CAD build for the part. Positions are in the model's coordinates, mm. Face numbers are marked on the shaded views. A direction names the side the tool comes from. Coordinates: 2 decimals unless noted, no trailing zeros. Write each loop counter-clockwise with the first axis right and the second up, starting at its lowest first coordinate (ties: lowest second). Pieces come first, ordered by that corner, then holes. Notation, with made-up numbers: (23, -30) - (29, -30) arc R28 ccw to (29, 2) - close; hole circle Ø11 at (26, 11). An arc over 180 degrees is marked (long way). One line per question, with ' | ' between items. Start each with the question number.
1. Two-plate mould, pull along Z, no slides. Class the marked faces 6, 7, 8 and 9: +Z half, -Z half, draft (parallel to the pull), parting line (faces both ways), or undercut.
2. Probe line 1 (Z direction, x = 0, y = -5); line 2 (Z direction, x = 0, y = -19.5); line 3 (Z direction, x = 0, y = -12.75). List the from-to ranges inside material, lowest first.
3. Band-saw the part on C-C, the plane y = -1.75. Write the cut outline in (x, z), then the cut area to 3 significant figures.
4. Band-saw the part on B-B, the plane y = -20. Write the cut outline in (x, z), then the cut area to 3 significant figures.
5. Band-saw the part on D-D, the plane z = 6. Write the cut outline in (x, y).
6. Flat gauge pins, fed straight in: P1, Ø4, axis at x = 1, y = -22.5, coming from the +Z side; P2, Ø9, axis at y = -5, z = 41.5, coming from the +X side; P3, Ø1.5, axis at x = -3.5, z = 36.5, coming from the -Y side. Where does each tip first touch, or does it go through?
7. Band-saw the part on A-A, the plane x = 0. Write the cut outline in (y, z), then the cut area to 3 significant figures.
8. Which spindle directions (+Z, -Z, +X, -X, +Y, -Y) get a long thin tool onto all of the face, cutting with end or side? Do the marked faces 1, 2, 3, 4 and 5. Say none if no direction does.
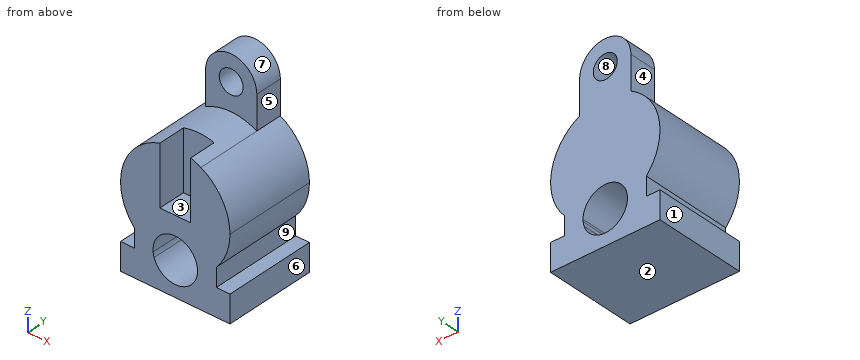
from build123d import *

# Parameters (mm, degrees)
F1_DEPTH = 27
F2_DEPTH = 8
F4_DEPTH = 8


with BuildPart() as f1:
    # F0 (on Front) → F1 (new body)
    with BuildSketch(Plane.XZ):
        with BuildLine():
            ThreePointArc((-7.5, 38.1332940251), (-15.7412312858, 26.8659444529), (-12, 13.4169947557))
            Line((-12, 13.4169947557), (-12, 22))
            Line((-12, 22), (12, 22))
            Line((12, 22), (12, 13.4169947557))
            ThreePointArc((12, 13.4169947557), (14.9666295471, 18.3431457505), (16, 24))
            ThreePointArc((16, 24), (13.7113092008, 32.2462112512), (7.5, 38.1332940251))
            Line((7.5, 38.1332940251), (-7.5, 38.1332940251))
        make_face()
        with BuildLine():
            Line((-12, 22), (-12, 13.4169947557))
            ThreePointArc((-12, 13.4169947557), (-9.454026078, 11.091809154), (-6.4690134152, 9.3660714286))
            ThreePointArc((-6.4690134152, 9.3660714286), (-0.3173427178, 16.4922487321), (6.5, 10))
            ThreePointArc((6.5, 10), (6.4922487321, 9.6826572822), (6.4690134152, 9.3660714286))
            ThreePointArc((6.4690134152, 9.3660714286), (9.454026078, 11.091809154), (12, 13.4169947557))
            Line((12, 13.4169947557), (12, 22))
            Line((12, 22), (-12, 22))
        make_face()
        with BuildLine():
            ThreePointArc((7.5, 38.1332940251), (0, 40), (-7.5, 38.1332940251))
            Line((-7.5, 38.1332940251), (7.5, 38.1332940251))
        make_face()
        with BuildLine():
            Line((-12, 8), (-16, 8))
            Line((-16, 8), (-16, 0))
            Line((-16, 0), (16, 0))
            Line((16, 0), (16, 8))
            Line((16, 8), (12, 8))
            Line((12, 8), (6.1846584384, 8))
            ThreePointArc((6.1846584384, 8), (0, 3.5), (-6.1846584384, 8))
            Line((-6.1846584384, 8), (-12, 8))
        make_face()
        with BuildLine():
            ThreePointArc((6.4690134152, 9.3660714286), (6.3635988742, 8.6753833128), (6.1846584384, 8))
            Line((6.1846584384, 8), (12, 8))
            Line((12, 8), (12, 13.4169947557))
            ThreePointArc((12, 13.4169947557), (9.454026078, 11.091809154), (6.4690134152, 9.3660714286))
        make_face()
        with BuildLine():
            Line((-12, 13.4169947557), (-12, 8))
            Line((-12, 8), (-6.1846584384, 8))
            ThreePointArc((-6.1846584384, 8), (-6.3635988742, 8.6753833128), (-6.4690134152, 9.3660714286))
            ThreePointArc((-6.4690134152, 9.3660714286), (-9.454026078, 11.091809154), (-12, 13.4169947557))
        make_face()
    extrude(amount=F1_DEPTH)

    # F0 (on Front) → F2 (join)
    with BuildSketch(Plane.XZ):
        with BuildLine():
            Line((-3.5, 48), (-7.5, 48))
            ThreePointArc((-7.5, 48), (0, 40.5), (7.5, 48))
            Line((7.5, 48), (3.5, 48))
            ThreePointArc((3.5, 48), (0, 44.5), (-3.5, 48))
        make_face()
        with BuildLine():
            ThreePointArc((7.5, 48), (0, 55.5), (-7.5, 48))
            Line((-7.5, 48), (-3.5, 48))
            ThreePointArc((-3.5, 48), (0, 51.5), (3.5, 48))
            Line((3.5, 48), (7.5, 48))
        make_face()
        with BuildLine():
            Line((-7.5, 48), (-7.5, 38.1332940251))
            ThreePointArc((-7.5, 38.1332940251), (0, 40), (7.5, 38.1332940251))
            Line((7.5, 38.1332940251), (7.5, 48))
            ThreePointArc((7.5, 48), (0, 40.5), (-7.5, 48))
        make_face()
    extrude(amount=F2_DEPTH)

    # F3 (on face) → F4 (cut)
    with BuildSketch(Plane.XZ.offset(27)):
        with BuildLine():
            Line((-4.5, 39.3541525328), (-4.5, 22))
            Line((-4.5, 22), (4.5, 22))
            Line((4.5, 22), (4.5, 39.3541525328))
            ThreePointArc((4.5, 39.3541525328), (0, 40), (-4.5, 39.3541525328))
        make_face()
    extrude(amount=-F4_DEPTH, mode=Mode.SUBTRACT)


solid = f1.part
Filled in:
1) face 6: draft | face 7: +Z half | face 8: undercut | face 9: undercut
2) line 1: z = 0 to 3.5, 16.5 to 44.5, 51.5 to 55.5 | line 2: z = 0 to 3.5, 16.5 to 22 | line 3: z = 0 to 3.5, 16.5 to 40
3) outline: (-16, 0) - (16, 0) - (16, 8) - (12, 8) - (12, 13.42) arc R16 ccw to (7.5, 38.13) - (7.5, 48) arc R7.5 ccw to (-7.5, 48) - (-7.5, 38.13) arc R16 ccw to (-12, 13.42) - (-12, 8) - (-16, 8) - close; hole circle Ø13 at (0, 10); hole circle Ø7 at (0, 48) | area: 1,150 mm²
4) outline: (-16, 0) - (16, 0) - (16, 8) - (12, 8) - (12, 13.42) arc R16 ccw to (4.5, 39.35) - (4.5, 22) - (-4.5, 22) - (-4.5, 39.35) arc R16 ccw to (-12, 13.42) - (-12, 8) - (-16, 8) - close; hole circle Ø13 at (0, 10) | area: 807 mm²
5) outline: (-16, -27) - (-5.12, -27) - (-5.12, 0) - (-16, 0) - close; (5.12, -27) - (16, -27) - (16, 0) - (5.12, 0) - close
6) P1: stops at z = 22 | P2: stops at x = 9.33 | P3: stops at y = -19
7) outline: (-27, 0) - (0, 0) - (0, 3.5) - (-27, 3.5) - close; (-27, 16.5) - (0, 16.5) - (0, 44.5) - (-8, 44.5) - (-8, 40) - (-19, 40) - (-19, 22) - (-27, 22) - close; (-8, 51.5) - (0, 51.5) - (0, 55.5) - (-8, 55.5) - close | area: 653 mm²
8) face 1: +Z, -Z, -X, +Y, -Y | face 2: -Z, +X, -X, +Y, -Y | face 3: +Z, -Y | face 4: +Z, -X, +Y, -Y | face 5: +Z, +X, +Y, -Y
